Part model, mm, in its own coordinate system. Give positions to 0.01 mm unless a question says otherwise; leave off trailing zeros. Order: outer loops, then holes, each group sorted by start corner. A loop starts at its lowest first (then second) coordinate and runs counter-clockwise, first axis right, second up.
1. Slice it at A-A on x = 0. List the corners of the cut face in (y, z), and give its area (3 significant figures).
2. Drop flat-ended pins along their axis: pin 1 Ø1 at (y, z) = (7.5, 1) entering from -X; pin 2 Ø1.5 at (y, z) = (43, 1.5) entering from +X; pin 3 Ø1.5 at (y, z) = (19.5, 2) entering from +X. Give the stop position or say it passes through.
3. Probe line 1 (Y direction, x = 0, z = 1.7); line 2 (Y direction, x = 3, z = 0.85); line 3 (Y direction, x = -1, z = 0.2). List the from-to ranges inside material, lowest first.
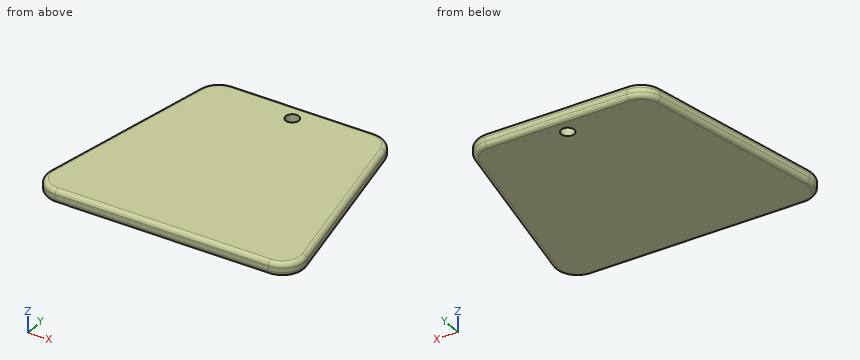
from build123d import *

# Parameters (mm, degrees)
F0_R     = 1.5
F1_DEPTH = 3
F2_R     = 5
F3_R     = 1


with BuildPart() as f1:
    # F0 (on Top) → F1 (new body)
    with BuildSketch(Plane.XY):
        Polygon((-30, 0), (0, 0), (30, 0), (20, 50), (0, 50), (-20, 50), align=None)
        with Locations((0, 45.908775)):
            Circle(F0_R, mode=Mode.SUBTRACT)
    extrude(amount=F1_DEPTH)

    # F2
    f2_edges = [f1.edges().sort_by_distance(p)[0] for p in [
        (-20, 50, 1.5),
        (20, 50, 1.5),
        (30, 0, 1.5),
        (-30, 0, 1.5),
    ]]
    fillet(f2_edges, radius=F2_R)

    # F3
    f3_edges = [f1.edges().sort_by_distance(p)[0] for p in [
        (24.803884, 25.980581, 3),
        (24.803884, 25.980581, 0),
    ]]
    fillet(f3_edges, radius=F3_R)


solid = f1.part
Data:
1. outline: (0, 1) arc R1 ccw to (1, 0) - (44.41, 0) - (44.41, 3) - (1, 3) arc R1 ccw to (0, 2) - close; (47.41, 0) - (49, 0) arc R1 ccw to (50, 1) - (50, 2) arc R1 ccw to (49, 3) - (47.41, 3) - close
1. area: 140 mm2
2. pin 1: stops at x = -28.6
2. pin 2: stops at x = 21.55
2. pin 3: stops at x = 26.25
3. line 1: y = 0 to 44.41, 47.41 to 50
3. line 2: y = 0.01 to 49.99
3. line 3: y = 0.4 to 44.79, 47.03 to 49.6
